The model under review builds one solid part; all positions refer to its coordinate system, in mm. A direction names the side the tool comes from. Coordinates: 2 decimals unless noted, no trailing zeros. Write each loop counter-clockwise with the first axis right and the second up, starting at its lowest first coordinate (ties: lowest second). Pieces come first, ordered by that corner, then holes. Notation, with made-up numbers: (-8, -15) -> (13, -15) arc R14 ccw to (13, 4) -> close; hole circle Ø3 at (51.5, -6.5). An arc over 180 degrees is marked (long way). Put each result on its own line as item: value. Start each with the question number.
from build123d import *

# Parameters (mm, degrees)
F0_R     = 12.5710937777
F1_DEPTH = 50.8


with BuildPart() as f1:
    # F0 (on Front) → F1 (new body)
    with BuildSketch(Plane.XZ):
        with BuildLine():
            Line((9.5049608148, 30.3477681373), (0, 31.8014356752))
            ThreePointArc((0, 31.8014356752), (-31.8014356752, 0), (0, -31.8014356752))
            Line((0, -31.8014356752), (9.4712928792, -30.3582924783))
            ThreePointArc((9.4712928792, -30.3582924783), (25.6176894183, -18.8431764804), (31.8014356752, 0))
            ThreePointArc((31.8014356752, 0), (25.6281360125, 18.8289658646), (9.5049608148, 30.3477681373))
        make_face()
        with BuildLine():
            ThreePointArc((-14.5709457578, 6.1619072221), (0, 15.8202895325), (14.5709457578, 6.1619072221))
            Line((14.5709457578, 6.1619072221), (20.2656146139, 6.1619072221))
            Line((20.2656146139, 6.1619072221), (20.2656146139, -7.6786847785))
            Line((20.2656146139, -7.6786847785), (13.8318242095, -7.6786847785))
            ThreePointArc((13.8318242095, -7.6786847785), (0, -15.8202895325), (-13.8318242095, -7.6786847785))
            Line((-13.8318242095, -7.6786847785), (-21.0093853861, -7.6786847785))
            Line((-21.0093853861, -7.6786847785), (-21.0093853861, 6.1619072221))
            Line((-21.0093853861, 6.1619072221), (-14.5709457578, 6.1619072221))
        make_face(mode=Mode.SUBTRACT)
        with BuildLine():
            Line((76.3308829682, 20.1275604352), (9.5049608148, 30.3477681373))
            ThreePointArc((9.5049608148, 30.3477681373), (25.6281360125, 18.8289658646), (31.8014356752, 0))
            ThreePointArc((31.8014356752, 0), (25.6176894183, -18.8431764804), (9.4712928792, -30.3582924783))
            Line((9.4712928792, -30.3582924783), (76.6803919445, -20.1176257266))
            ThreePointArc((76.6803919445, -20.1176257266), (55.8029369519, -0.1748250718), (76.3308829682, 20.1275604352))
        make_face()
        with BuildLine():
            ThreePointArc((96.0651373404, 0), (90.3085177912, 14.0939657718), (76.3308829682, 20.1275604352))
            ThreePointArc((76.3308829682, 20.1275604352), (55.8029369519, -0.1748250718), (76.6803919445, -20.1176257266))
            ThreePointArc((76.6803919445, -20.1176257266), (90.4303700533, -13.9686006721), (96.0651373404, 0))
        make_face()
        with Locations((75.9336575866, 0)):
            Circle(F0_R, mode=Mode.SUBTRACT)
    extrude(amount=F1_DEPTH)


solid = f1.part
1. Consider section B-B on x = 4. State the section outline as (y, z) points, then the cut area to 3 significant figures.
2. Wall thickness on line 1 (X direction, y = -16, z = -7.5); line 2 (X direction, y = -7.5, z = 6); line 3 (Z direction, x = -9.5, y = -38): over which ranges is each line inside the solid? List them lowest first. Write a range as from..to.
3. The part is to be moulded in two halves that separate along X. For faces 1 (the cylindrical face through (-31.794, -25.044, 0.699)), 2 (the flat face through (31, 0, 0)), 3 (the flat face through (17, -25, -7.679)), say which applies: released by +X, released by -X, zero draft, split by the parting line, or undercut.
4. Insertion check: P1, Ø3, axis at x = 16.5, y = -18.5, coming from the -Z side; P2, Ø12, axis at y = -33, z = -7.5, coming from the -X side; P3, Ø5, axis at x = 72.5, y = -30, coming from the -Z side; P4, Ø1, axis at x = -17.5, z = 6.5, coming from the +Y side. Each pin has a flat end and moves straight along its axis. Give the tip position at first contact, or say it passes through.
5. Consider section C-C on x = 83. State the section outline as (y, z) points.
6. Consider section D-D on z = -27. State the section outline as (x, y) points, then the cut area to 3 significant figures.
7. Consider section A-A on y = -38. State the section outline as (x, z) points.
8. Tool access review of faces 4 (the flat face through (31, -50.8, 0)), 5 (the flat face through (-18, -25, 6.162)): name each direction out of +Z, -Z, +X, -X, +Y, -Y from which nothing blocks a thin tool from reaching the whole face with its end or side.
Output values:
1. outline: (-50.8, -31.19) -> (0, -31.19) -> (0, -15.31) -> (-50.8, -15.31) -> close; (-50.8, 15.31) -> (0, 15.31) -> (0, 31.19) -> (-50.8, 31.19) -> close
1. area: 1,610 mm^2
2. line 1: x = -30.9..-21.01, 20.27..65.84, 86.02..94.62
2. line 2: x = -31.23..-21.01, 20.27..64.89, 86.98..95.15
2. line 3: z = -30.35..-12.65, 12.65..30.35
3. face 1: released by -X
3. face 2: zero draft
3. face 3: undercut
4. P1: stops at z = -29.52
4. P2: stops at x = -31.77
4. P3: stops at z = -21.14
4. P4: stops at y = 0
5. outline: (-50.8, -18.85) -> (0, -18.85) -> (0, -10.4) -> (-50.8, -10.4) -> close; (-50.8, 10.4) -> (0, 10.4) -> (0, 18.85) -> (-50.8, 18.85) -> close
6. outline: (-16.8, -50.8) -> (31.51, -50.8) -> (31.51, 0) -> (-16.8, 0) -> close
6. area: 2,450 mm^2
7. outline: (0, -31.8) -> (76.68, -20.12) arc R20.13 ccw to (76.33, 20.13) -> (0, 31.8) arc R31.8 ccw to start; hole (-21.01, -7.68) -> (-13.83, -7.68) arc R15.82 ccw to (13.83, -7.68) -> (20.27, -7.68) -> (20.27, 6.16) -> (14.57, 6.16) arc R15.82 ccw to (-14.57, 6.16) -> (-21.01, 6.16) -> close; hole circle Ø25.14 at (75.93, 0)
8. face 4: +Z, -Z, +X, -X, -Y
8. face 5: +Y, -Y
